Autodesk Inventor part; units mm, degrees
ref_plane "YZ Plane" through (0, 0, 0) normal (1, 0, 0) x (0, 1, 0)
ref_plane "XZ Plane" through (0, 0, 0) normal (0, 1, 0) x (-1, 0, 0)
ref_plane "XY Plane" through (0, 0, 0) normal (0, 0, 1) x (1, 0, 0)
sketch "Sketch1" plane through (0, 0, 0) normal (0, 1, 0) x (-1, 0, 0)
  line L0 (0, 0) -> (762, 0)
  line L1 (762, 0) -> (762, 762)
  line L2 (762, 762) -> (0, 762)
  line L3 (0, 762) -> (0, 0)
  line L4 (0, 0) -> (190.5, 0)
  line L5 (190.5, 0) -> (190.5, 69.85)
  line L6 (190.5, 69.85) -> (0, 69.85)
  line L7 (0, 69.85) -> (0, 0)
  line L8 (0, 0) -> (69.85, 0)
  line L9 (69.85, 0) -> (69.85, 190.5)
  line L10 (69.85, 190.5) -> (0, 190.5)
  line L11 (0, 190.5) -> (0, 0)
  line L12 (69.85, 190.5) -> (190.5, 69.85)
  line L13 (381, 0) -> (381, 762)
  line L14 (0, 381) -> (762, 381)
  line L15 (190.5, 762) -> (190.5, 692.15)
  line L16 (190.5, 692.15) -> (0, 692.15)
  line L17 (69.85, 762) -> (69.85, 571.5)
  line L18 (69.85, 571.5) -> (0, 571.5)
  line L19 (69.85, 571.5) -> (190.5, 692.15)
  line L20 (571.5, 0) -> (571.5, 69.85)
  line L21 (571.5, 69.85) -> (762, 69.85)
  line L22 (692.15, 0) -> (692.15, 190.5)
  line L23 (692.15, 190.5) -> (762, 190.5)
  line L24 (692.15, 190.5) -> (571.5, 69.85)
  line L25 (571.5, 692.15) -> (762, 692.15)
  line L26 (692.15, 571.5) -> (571.5, 692.15)
  line L27 (692.15, 762) -> (692.15, 571.5)
  line L28 (571.5, 762) -> (571.5, 692.15)
  line L29 (692.15, 571.5) -> (762, 571.5)
  circle A0 centre (749.3, 749.3) radius 2.3812
  circle A1 centre (749.3, 723.9) radius 2.3812
  circle A2 centre (749.3, 698.5) radius 2.3812
  circle A3 centre (749.3, 673.1) radius 2.3812
  circle A4 centre (749.3, 647.7) radius 2.3812
  circle A5 centre (749.3, 622.3) radius 2.3812
  circle A6 centre (749.3, 596.9) radius 2.3812
  circle A7 centre (749.3, 571.5) radius 2.3812
  circle A8 centre (749.3, 546.1) radius 2.3812
  circle A9 centre (749.3, 520.7) radius 2.3812
  circle A10 centre (749.3, 495.3) radius 2.3812
  circle A11 centre (749.3, 469.9) radius 2.3812
  circle A12 centre (749.3, 444.5) radius 2.3812
  circle A13 centre (749.3, 419.1) radius 2.3812
  circle A14 centre (749.3, 393.7) radius 2.3812
  circle A15 centre (749.3, 368.3) radius 2.3812
  circle A16 centre (749.3, 342.9) radius 2.3812
  circle A17 centre (749.3, 317.5) radius 2.3812
  circle A18 centre (749.3, 292.1) radius 2.3812
  circle A19 centre (749.3, 266.7) radius 2.3812
  circle A20 centre (749.3, 241.3) radius 2.3812
  circle A21 centre (749.3, 215.9) radius 2.3812
  circle A22 centre (749.3, 190.5) radius 2.3812
  circle A23 centre (749.3, 165.1) radius 2.3812
  circle A24 centre (749.3, 139.7) radius 2.3812
  circle A25 centre (749.3, 114.3) radius 2.3812
  circle A26 centre (749.3, 88.9) radius 2.3812
  circle A27 centre (749.3, 63.5) radius 2.3812
  circle A28 centre (749.3, 38.1) radius 2.3812
  circle A29 centre (749.3, 12.7) radius 2.3812
  circle A30 centre (12.7, 749.3) radius 2.3812
  circle A31 centre (12.7, 723.9) radius 2.3812
  circle A32 centre (12.7, 698.5) radius 2.3812
  circle A33 centre (12.7, 673.1) radius 2.3812
  circle A34 centre (12.7, 647.7) radius 2.3812
  circle A35 centre (12.7, 622.3) radius 2.3812
  circle A36 centre (12.7, 596.9) radius 2.3812
  circle A37 centre (12.7, 571.5) radius 2.3812
  circle A38 centre (12.7, 546.1) radius 2.3812
  circle A39 centre (12.7, 520.7) radius 2.3812
  circle A40 centre (12.7, 495.3) radius 2.3812
  circle A41 centre (12.7, 469.9) radius 2.3812
  circle A42 centre (12.7, 444.5) radius 2.3812
  circle A43 centre (12.7, 419.1) radius 2.3812
  circle A44 centre (12.7, 393.7) radius 2.3812
  circle A45 centre (12.7, 368.3) radius 2.3812
  circle A46 centre (12.7, 342.9) radius 2.3812
  circle A47 centre (12.7, 317.5) radius 2.3812
  circle A48 centre (12.7, 292.1) radius 2.3812
  circle A49 centre (12.7, 266.7) radius 2.3812
  circle A50 centre (12.7, 241.3) radius 2.3812
  circle A51 centre (12.7, 215.9) radius 2.3812
  circle A52 centre (12.7, 190.5) radius 2.3812
  circle A53 centre (12.7, 165.1) radius 2.3812
  circle A54 centre (12.7, 139.7) radius 2.3812
  circle A55 centre (12.7, 114.3) radius 2.3812
  circle A56 centre (12.7, 88.9) radius 2.3812
  circle A57 centre (12.7, 63.5) radius 2.3812
  circle A58 centre (12.7, 38.1) radius 2.3812
  circle A59 centre (12.7, 12.7) radius 2.3812
  circle A60 centre (723.9, 749.3) radius 2.3812
  circle A61 centre (698.5, 749.3) radius 2.3812
  circle A62 centre (673.1, 749.3) radius 2.3812
  circle A63 centre (647.7, 749.3) radius 2.3812
  circle A64 centre (622.3, 749.3) radius 2.3812
  circle A65 centre (596.9, 749.3) radius 2.3812
  circle A66 centre (571.5, 749.3) radius 2.3812
  circle A67 centre (546.1, 749.3) radius 2.3812
  circle A68 centre (520.7, 749.3) radius 2.3812
  circle A69 centre (495.3, 749.3) radius 2.3812
  circle A70 centre (469.9, 749.3) radius 2.3812
  circle A71 centre (444.5, 749.3) radius 2.3812
  circle A72 centre (419.1, 749.3) radius 2.3812
  circle A73 centre (393.7, 749.3) radius 2.3812
  circle A74 centre (368.3, 749.3) radius 2.3812
  circle A75 centre (342.9, 749.3) radius 2.3812
  circle A76 centre (317.5, 749.3) radius 2.3812
  circle A77 centre (292.1, 749.3) radius 2.3812
  circle A78 centre (266.7, 749.3) radius 2.3812
  circle A79 centre (241.3, 749.3) radius 2.3812
  circle A80 centre (215.9, 749.3) radius 2.3812
  circle A81 centre (190.5, 749.3) radius 2.3812
  circle A82 centre (165.1, 749.3) radius 2.3812
  circle A83 centre (139.7, 749.3) radius 2.3812
  circle A84 centre (114.3, 749.3) radius 2.3812
  circle A85 centre (88.9, 749.3) radius 2.3812
  circle A86 centre (63.5, 749.3) radius 2.3812
  circle A87 centre (38.1, 749.3) radius 2.3812
  circle A88 centre (12.7, 749.3) radius 2.3812
  circle A89 centre (749.3, 12.7) radius 2.3812
  circle A90 centre (723.9, 12.7) radius 2.3812
  circle A91 centre (698.5, 12.7) radius 2.3812
  circle A92 centre (673.1, 12.7) radius 2.3812
  circle A93 centre (647.7, 12.7) radius 2.3812
  circle A94 centre (622.3, 12.7) radius 2.3812
  circle A95 centre (596.9, 12.7) radius 2.3812
  circle A96 centre (571.5, 12.7) radius 2.3812
  circle A97 centre (546.1, 12.7) radius 2.3812
  circle A98 centre (520.7, 12.7) radius 2.3812
  circle A99 centre (495.3, 12.7) radius 2.3812
  circle A100 centre (469.9, 12.7) radius 2.3812
  circle A101 centre (444.5, 12.7) radius 2.3812
  circle A102 centre (419.1, 12.7) radius 2.3812
  circle A103 centre (393.7, 12.7) radius 2.3812
  circle A104 centre (368.3, 12.7) radius 2.3812
  circle A105 centre (342.9, 12.7) radius 2.3812
  circle A106 centre (317.5, 12.7) radius 2.3812
  circle A107 centre (292.1, 12.7) radius 2.3812
  circle A108 centre (266.7, 12.7) radius 2.3812
  circle A109 centre (241.3, 12.7) radius 2.3812
  circle A110 centre (215.9, 12.7) radius 2.3812
  circle A111 centre (190.5, 12.7) radius 2.3812
  circle A112 centre (165.1, 12.7) radius 2.3812
  circle A113 centre (139.7, 12.7) radius 2.3812
  circle A114 centre (114.3, 12.7) radius 2.3812
  circle A115 centre (88.9, 12.7) radius 2.3812
  circle A116 centre (63.5, 12.7) radius 2.3812
  circle A117 centre (38.1, 12.7) radius 2.3812
  circle A118 centre (12.7, 12.7) radius 2.3812
  dimension "d0" = 762
  dimension "d1" = 762
  dimension "d2" = 190.5
  dimension "d3" = 69.85
  dimension "d4" = 69.85
  dimension "d5" = 190.5
  dimension "d29" = 12.7
  dimension "d30" = 12.7
  dimension "d31" = 4.7625
  dimension "d34" = 25.4
  dimension "d37" = 736.6
  dimension "d42" = 25.4
  dimension "d45" = 736.6
extrude "Extrusion1" add sketch "Sketch1" along normal blind 3.175 contours L5 A111 L12 L10 A52 L3 L14 L13 L0 | L13 L14 L1 L23 A22 L24 L20 A96 L0 | L5 A111 | L3 L18 A37 L19 L15 A81 L2 L13 L14 | A52 L10 | L13 L2 L28 A66 L26 L29 A7 L1 L14 | A96 L20 | L18 A37 | L28 A66 | A81 L15 | L23 A22 | A7 L29 picked at (191.2937, 12.7) picked at (13.1509, 191.1532) picked at (570.7578, 12.4185) picked at (12.2491, 570.8468) picked at (570.7578, 749.5815) picked at (191.6271, 749.4766) picked at (749.3957, 191.6679) picked at (749.5815, 570.7578)
properties part number "Base Plate V1.2"
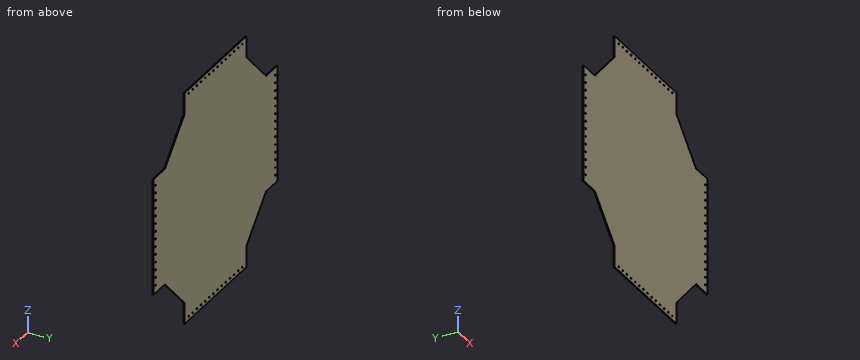
The model under review builds one solid part; all positions refer to its coordinate system, in mm. Round coordinates to 2 decimals unless told otherwise and drop trailing zeros. Loops run counter-clockwise (first coordinate to the right, second up) from the corner with the lowest first, then second, coordinate; pieces in that order, holes last. Notation, with made-up numbers: (-31, 41) -> (22, 41) arc R10 cw to (22, 54) -> close; hole circle Ø4 at (-26.5, 79.5). An arc over 180 degrees is marked (long way). One line per question, with ' | ' between items. Start each with the question number.
Item 1: Add section C-C, the plane z = 100. Write out the cut boundary in (x, y) (3 decimals), then the cut area to 3 significant figures.
Item 2: For pin 1 (7.5 mm diameter, centred on x = -368.3, z = 12.7, fed in from +Y) (3 decimals); pin 2 (1 mm diameter, centred on x = -725.5, y = 1.5, fed in from +Z); pin 3 (1.6 mm diameter, centred on x = -36.5, y = 2, fed in from -Z); pin 4 (1 mm diameter, centred on y = 1, z = 28.5, fed in from -X), all flat-tipped, find the tip position at first contact; note any pin that passes through.
Item 3: Add section A-A, the plane y = 1.3. Count the separate pieces of the cut face and the enclosed holes in it, then the cut area to 3 significant figures.
Item 4: Add section B-B, the plane x = -709.5. Write out the cut boundary in (y, z) (3 decimals), then the cut area to 3 significant figures.
Item 5: Wall thickness on line 1 along Z through (x, y) = (-495.3, 1.15); line 2 along X through (y, z) = (2.4, 393); line 3 along Z through (x, y) = (-215, 1.15): over which ranges is each line inside the solid? List them lowest first. Write a range as [from, to].
Return value:
1) outline: (-601.65, 0) -> (-160.35, 0) -> (-160.35, 3.175) -> (-601.65, 3.175) -> close | area: 1,400 mm2
2) pin 1: stops at y = 3.175 | pin 2: stops at z = 571.5 | pin 3: stops at z = 190.5 | pin 4: stops at x = -571.5
3) separate pieces: 1 | enclosed holes: 56 | area: 464,000 mm2
4) outline: (0, 190.5) -> (3.175, 190.5) -> (3.175, 571.5) -> (0, 571.5) -> close | area: 1,210 mm2
5) line 1: z = [0, 10.32], [15.08, 746.92], [751.68, 762] | line 2: x = [-762, -751.58], [-747.02, -14.98], [-10.42, 0] | line 3: z = [0, 10.5], [14.9, 747.1], [751.5, 762]
